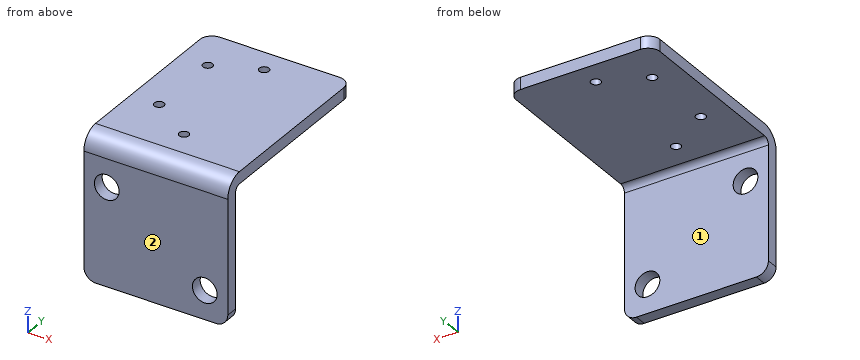
```python
from build123d import *

# Parameters (mm, degrees)
BASE_FLANGE1_DEPTH = 76.2
SKETCH3_R          = 6.5405
TAB1_DEPTH         = 6.35
SKETCH3_2_R        = 6.5405
CUT_EXTRUDE1_DEPTH = 12.7
SKETCH4_R          = 2.5527
CUT_EXTRUDE2_DEPTH = 12.7
FILLET1_R          = 6.35


# Sheet-metal steps are written as plain solids
with BuildPart() as part:
    # Sketch1 → Base-Flange1 (new body)
    with BuildSketch(Plane(origin=(0, 0, 0), x_dir=(0, 0, -1), z_dir=(1, 0, 0))):
        with BuildLine():
            Line((76.2, 0), (9.525, 0))
            ThreePointArc((9.525, 0), (2.789807909, 2.789807909), (0, 9.525))
            Line((0, 9.525), (0, 101.6))
            Line((0, 101.6), (6.35, 101.6))
            Line((6.35, 101.6), (6.35, 9.525))
            ThreePointArc((6.35, 9.525), (7.27993597, 7.27993597), (9.525, 6.35))
            Line((9.525, 6.35), (76.2, 6.35))
            Line((76.2, 6.35), (76.2, 0))
        make_face()
    extrude(amount=BASE_FLANGE1_DEPTH)

    # Sketch3 → Tab1 (add)
    with BuildSketch(Plane(origin=(0, 6.35, 0), x_dir=(-1, 0, 0), z_dir=(0, 1, 0))):
        with Locations((-12.1158, -24.384)):
            Circle(SKETCH3_R)
        with Locations((-64.008, -60.96)):
            Circle(SKETCH3_R)
    extrude(amount=-TAB1_DEPTH)

    # Sketch3<2> → Cut-Extrude1 (cut)
    with BuildSketch(Plane(origin=(0, 6.35, 0), x_dir=(-1, 0, 0), z_dir=(0, 1, 0))):
        with Locations(Location((-12.1158, -24.384, 0), (0, 0, 90))):
            Circle(SKETCH3_2_R)
        with Locations(Location((-64.008, -60.96, 0), (0, 0, 90))):
            Circle(SKETCH3_2_R)
    extrude(amount=-CUT_EXTRUDE1_DEPTH, mode=Mode.SUBTRACT)

    # Sketch4 → Cut-Extrude2 (cut)
    with BuildSketch(Plane(origin=(0, 0, -6.35), x_dir=(-1, 0, 0), z_dir=(0, 0, -1))):
        with Locations((-38.1, 88.9)):
            Circle(SKETCH4_R)
        with Locations((-38.1, 23.114)):
            Circle(SKETCH4_R)
        with Locations((-14.986, 78.486)):
            Circle(SKETCH4_R)
        with Locations((-14.986, 38.608)):
            Circle(SKETCH4_R)
    extrude(amount=-CUT_EXTRUDE2_DEPTH, mode=Mode.SUBTRACT)

    # Fillet1
    fillet1_edges = [part.edges().sort_by_distance(p)[0] for p in [
        (76.2, 101.6, -3.175),
        (0, 101.6, -3.175),
        (76.2, 3.175, -76.2),
        (0, 3.175, -76.2),
    ]]
    fillet(fillet1_edges, radius=FILLET1_R)


solid = part.part
```
CAD build for the part. Positions are in the model's coordinates, mm. Face numbers are marked on the shaded views. A direction names the side the tool comes from. Coordinates: 2 decimals unless noted, no trailing zeros. Write each loop counter-clockwise with the first axis right and the second up, starting at its lowest first coordinate (ties: lowest second). Pieces come first, ordered by that corner, then holes.
(1) Cut at C-C, the plane z = -60.96. List the corners of the cut face in (x, y).
(2) Cut at D-D, the plane x = 50.5. List the corners of the cut face in (y, z) (3 decimals).
(3) Flat gauge pins, fed straight in: pin 1 (10 mm diameter, centred on x = 31, y = 40, fed in from -Z); pin 2 (1 mm diameter, centred on x = 9.5, z = -17, fed in from +Y). Where does each tip first touch, or does it go through?
(4) Drill centre lines: probe 1 along Z at (x, y) = (14, 13); probe 2 along Y at (x, z) = (22.5, -13); probe 3 along X at (y, z) = (87, -3.5). Where is each one in solid material? Low to high.
(5) 3-axis set-ups, long thin cutter, end or side, ignore diameter. For the marked faces 1 and 2: which of +Z, -Z, +X, -X, +Y, -Y reach the whole face in a straight line?
(6) Cut at B-B, the plane x = 38.1. List the corners of the cut face in (y, z) (3 decimals), and give its area (3 significant figures).
(7) Cut at A-A, the plane y = 88.9. List the corners of the cut face in (x, z), and give its area (3 significant figures).
Geometry says:
1. outline: (0, 0) - (57.47, 0) - (57.47, 6.35) - (0, 6.35) - close; (70.55, 0) - (76.2, 0) - (76.2, 6.35) - (70.55, 6.35) - close
2. outline: (0, -76.2) - (6.35, -76.2) - (6.35, -9.525) arc R3.175 cw to (9.525, -6.35) - (101.6, -6.35) - (101.6, 0) - (9.525, 0) arc R9.525 ccw to (0, -9.525) - close
3. pin 1: stops at z = -6.35
3. pin 2: stops at y = 6.35
4. probe 1: z = -6.35 to 0
4. probe 2: y = 0 to 6.35
4. probe 3: x = 0 to 36.4, 39.8 to 76.2
5. face 1: -Z, +X, -X, +Y
5. face 2: +Z, -Z, +X, -X, -Y
6. outline: (0, -76.2) - (6.35, -76.2) - (6.35, -9.525) arc R3.175 cw to (9.525, -6.35) - (20.561, -6.35) - (20.561, 0) - (9.525, 0) arc R9.525 ccw to (0, -9.525) - close; (25.667, -6.35) - (86.347, -6.35) - (86.347, 0) - (25.667, 0) - close; (91.453, -6.35) - (101.6, -6.35) - (101.6, 0) - (91.453, 0) - close
6. area: 1,010 mm2
7. outline: (0, -6.35) - (35.55, -6.35) - (35.55, 0) - (0, 0) - close; (40.65, -6.35) - (76.2, -6.35) - (76.2, 0) - (40.65, 0) - close
7. area: 451 mm2
